Could you check a few things on this drawing? It's one solid part, dimensions in mm from its lowest x, y, z. A direction names the side the tool comes from. Round coordinates to 2 decimals unless told otherwise and drop trailing zeros. Loops run counter-clockwise (first coordinate to the right, second up) from the corner with the lowest first, then second, coordinate; pieces in that order, holes last.
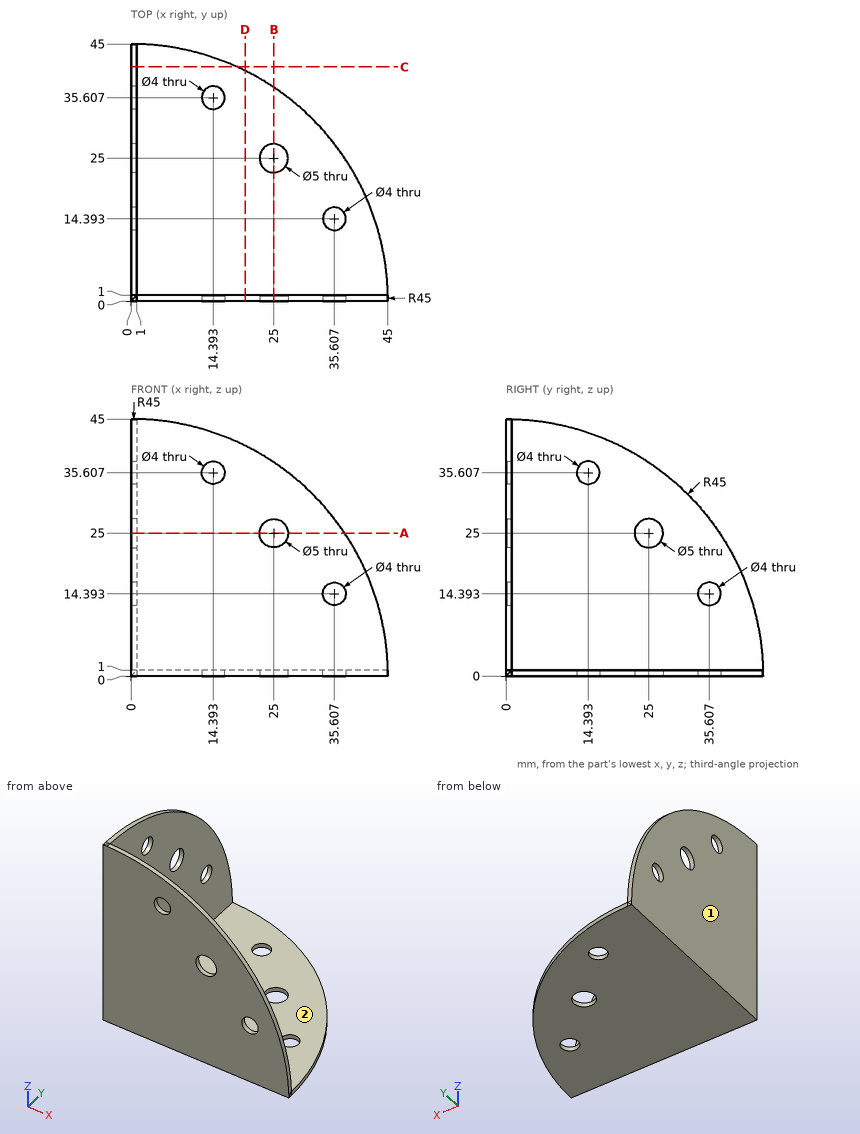
(1) Suppose I cut it at A-A (z = 25). Write out the boundary of the cut face in (x, y).
(2) Suppose I cut it at C-C (y = 41). Write out the boundary of the cut face in (x, z).
(3) For pin 1 (3 mm diameter, centred on y = 25.5, z = 16.5, fed in from +X); pin 2 (4 mm diameter, centred on x = 25.5, y = 20, fed in from +Z); pin 3 (1.5 mm diameter, centred on x = 19.5, z = 28.5, fed in from +Y), each with a flat end and sliding along its axis, tell me the tip position at first contact or that it passes through.
(4) Which directions (+Z, -Z, +X, -X, +Y, -Y) give clear straight access to the entire face, cutting with the end or side of a thin tool? Please do the marked faces 1 and 2.
(5) If I drill on line 1 (Z direction, x = 13.5, y = 8), over which ranges is the centre line in solid material (lowest first)?
(6) Suppose I cut it at D-D (x = 20). Write out the boundary of the cut face in (y, z).
Check result:
1. outline: (0, 0) - (22.5, 0) - (22.5, 1) - (1, 1) - (1, 22.5) - (0, 22.5) - close; (0, 27.5) - (1, 27.5) - (1, 37.42) - (0, 37.42) - close; (27.5, 0) - (37.42, 0) - (37.42, 1) - (27.5, 1) - close
2. outline: (0, 0) - (18.55, 0) - (18.55, 1) - (1, 1) - (1, 18.55) - (0, 18.55) - close
3. pin 1: stops at x = 1
3. pin 2: stops at z = 1
3. pin 3: stops at y = 1
4. face 1: +Z, -Z, -X, +Y, -Y
4. face 2: +Z, +X, +Y
5. line 1: z = 0 to 1
6. outline: (0, 0) - (40.31, 0) - (40.31, 1) - (1, 1) - (1, 40.31) - (0, 40.31) - close
